```python
from build123d import *

# Parameters (mm, degrees)
F1_DEPTH = 19.558
F2_T     = -2.54
F3_START = 7.62
F3_DEPTH = 4.572
F4_START = 7.112
F4_DEPTH = 5.08
F5_START = 7.366
F5_DEPTH = 4.699


with BuildPart() as f1:
    # F0 (on Front) → F1 (new body)
    with BuildSketch(Plane.XZ):
        with BuildLine():
            Line((10.5598789448, -0.6324698916), (10.4941550919, 1.3355786754))
            ThreePointArc((10.4941550919, 1.3355786754), (-10.5729083556, -0.3530869534), (10.5598789448, -0.6324698916))
        make_face()
        with BuildLine():
            ThreePointArc((10.5598789448, -0.6324698916), (10.574070523, -0.3163764621), (10.5788024602, 0))
            ThreePointArc((10.5788024602, 0), (10.5576194096, 0.6691292056), (10.4941550919, 1.3355786754))
            Line((10.4941550919, 1.3355786754), (10.5598789448, -0.6324698916))
        make_face()
    extrude(amount=F1_DEPTH)

    # F2
    f2_openings = [f1.faces().sort_by_distance(p)[0] for p in [
        (0, -19.558, 0),
    ]]
    offset(amount=F2_T, openings=f2_openings)

    # F0 (on Front) → F3 (join)
    with BuildSketch(Plane.XZ.offset(F3_START)):
        with BuildLine():
            ThreePointArc((10.4941550919, 1.3355786754), (10.5576194096, 0.6691292056), (10.5788024602, 0))
            ThreePointArc((10.5788024602, 0), (10.574070523, -0.3163764621), (10.5598789448, -0.6324698916))
            Line((10.5598789448, -0.6324698916), (47.8745400906, -0.6324698916))
            Line((47.8745400906, -0.6324698916), (47.8745400906, 1.3355786754))
            Line((47.8745400906, 1.3355786754), (10.4941550919, 1.3355786754))
        make_face()
    extrude(amount=F3_DEPTH)

    # F0 (on Front) → F4 (join)
    with BuildSketch(Plane.XZ.offset(F4_START)):
        Polygon((47.8745400906, 6.7476513796), (47.8745400906, 1.3355786754), (47.8745400906, -0.6324698916), (47.8745400906, -7.1075903252), (58.2372918725, -7.1075903252), (65.9249648452, -4.9262144603), (58.2372918725, -3.502572421), (65.9249648452, -1.8891115906), (58.2372918725, 0), (65.9249648452, 1.1479911627), (58.2372918725, 3.6156391725), (65.9249648452, 5.7036471553), (58.2372918725, 6.7476513796), align=None)
        with BuildLine():
            ThreePointArc((53.0559159815, 3.2301100822), (56.5529149026, -0.3554173745), (53.0559159815, -3.9409448312))
            Line((53.0559159815, -3.9409448312), (53.0559159815, -1.589890453))
            Line((53.0559159815, -1.589890453), (53.0559159815, 0.9286483983))
            Line((53.0559159815, 0.9286483983), (53.0559159815, 3.2301100822))
        make_face(mode=Mode.SUBTRACT)
    extrude(amount=F4_DEPTH)

    # F0 (on Front) → F5 (join)
    with BuildSketch(Plane.XZ.offset(F5_START)):
        with BuildLine():
            Line((53.0559159815, 0.9286483983), (53.0559159815, -1.589890453))
            ThreePointArc((53.0559159815, -1.589890453), (54.3151854072, -0.3306210274), (53.0559159815, 0.9286483983))
        make_face()
    extrude(amount=F5_DEPTH)


solid = f1.part
```
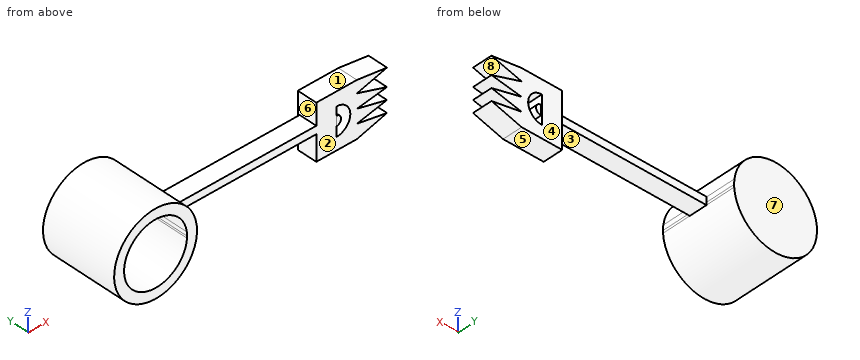
CAD build for the part. Positions are in the model's coordinates, mm. Face numbers are marked on the shaded views. A direction names the side the tool comes from. Give positions to 0.01 mm unless a question says otherwise; leave off trailing zeros. Loops run counter-clockwise (first coordinate to the right, second up) from the corner with the lowest first, then second, coordinate; pieces in that order, holes last. Notation, with made-up numbers: (41, 29) -> (66, 29) arc R18 cw to (66, 50) -> close; hole circle Ø11 at (16.25, -13.75). An arc over 180 degrees is marked (long way). Use a Markdown table: item, result.
1. Slice it at A-A (z = -6). List the corners of the cut face in (x, y).
Check result:
| item | result |
|---|---|
| outline | (-8.71, -19.56) -> (-5.35, -19.56) -> (-5.35, -2.54) -> (5.35, -2.54) -> (5.35, -19.56) -> (8.71, -19.56) -> (8.71, 0) -> (-8.71, 0) -> close; (47.87, -12.19) -> (62.14, -12.19) -> (62.14, -7.11) -> (47.87, -7.11) -> close |
2. Mould opens along X. For the marked faces 6, 7 and 8 say: pulls with the +X half, pulls with the -X half, needs draft (parallel to the pull), parting line crosses it, or undercut.
Check result:
| item | result |
|---|---|
| face 6 | undercut |
| face 7 | needs draft |
| face 8 | pulls with the +X half |
3. Flat gauge pins, fed straight in: pin 1 (6 mm diameter, centred on y = -13.5, z = 5.5, fed in from -X); pin 2 (11 mm diameter, centred on x = 59.5, z = 0, fed in from +Y); pin 3 (3 mm diameter, centred on y = -15.5, z = 2.5, fed in from +X); pin 4 (5.5 mm diameter, centred on y = -10, z = 1.5, fed in from -X). Where does each tip first touch, or does it go through?
Check result:
| item | result |
|---|---|
| pin 1 | stops at x = -10.28 |
| pin 2 | stops at y = -7.11 |
| pin 3 | stops at x = 10.53 |
| pin 4 | stops at x = -10.58 |
4. Slice it at B-B (y = -15). List the corners of the cut face in (x, z).
Check result:
| item | result |
|---|---|
| outline | circle Ø21.16 at (0, 0); hole circle Ø16.08 at (0, 0) |
5. Slice it at D-D (z = 4.75). List the corners of the cut face in (x, y).
Check result:
| item | result |
|---|---|
| outline | (-9.45, -19.56) -> (-6.49, -19.56) -> (-6.49, -2.54) -> (6.49, -2.54) -> (6.49, -19.56) -> (9.45, -19.56) -> (9.45, 0) -> (-9.45, 0) -> close; (47.87, -12.19) -> (62.41, -12.19) -> (62.41, -7.11) -> (47.87, -7.11) -> close |
6. Slice it at C-C (x = 0). List the corners of the cut face in (y, z).
Check result:
| item | result |
|---|---|
| outline | (-19.56, -10.58) -> (0, -10.58) -> (0, 10.58) -> (-19.56, 10.58) -> (-19.56, 8.04) -> (-2.54, 8.04) -> (-2.54, -8.04) -> (-19.56, -8.04) -> close |
7. Wall check: L1, parallel to Z at x = 0, y = -12.75; L2, parallel to X at y = -18.25, z = -0.25; L3, parallel to Z at x = 53, y = -11. Give the ranges that are in metal, low to high. Write a range as [from, to].
Check result:
| item | result |
|---|---|
| L1 | z = [-10.58, -8.04], [8.04, 10.58] |
| L2 | x = [-10.58, -8.03], [8.03, 10.58] |
| L3 | z = [-7.11, 6.75] |
8. Which spindle directions (+Z, -Z, +X, -X, +Y, -Y) get a long thin tool onto all of the face, cutting with end or side? Do the marked faces 1, 2, 3, 4 and 5. Say none if no direction does.
Check result:
| item | result |
|---|---|
| face 1 | +Z, +X, +Y, -Y |
| face 2 | +Z, -Z, +X, -Y |
| face 3 | -Z, +Y, -Y |
| face 4 | +Z, -Z, +X, +Y |
| face 5 | -Z, +X, +Y, -Y |
